from build123d import *

# Parameters (mm, degrees)
F0_W      = 58.45
F0_H      = 12.7
F1_DEPTH  = 2.5
F2_W      = 58.45
F2_H      = 1.21
F6_DEPTH  = 0.6
F4_W      = 58.45
F4_H      = 1.21
F7_DEPTH  = 0.6
F5_W      = 1.21
F5_H      = 12.7
F8_DEPTH  = 0.6
F3_W      = 1.21
F3_H      = 12.7
F9_DEPTH  = 0.6
F10_W     = 3.2
F10_H     = 8.5
F11_DEPTH = 1
F12_R     = 2.4
F14_W     = 4.5
F14_H     = 8.5
F13_W     = 4.5
F13_H     = 8.5
F15_DEPTH = 13.25
F16_R     = 2.24999
F17_R     = 3.15
F18_DEPTH = 16.751


# Not quite as in the source:
# - a fillet or chamfer is up to 0.001 mm smaller than in the source, because OpenCascade refuses the exact size


with BuildPart() as f1:
    # F0 (on Front) → F1 (new body)
    with BuildSketch(Plane.XZ):
        Rectangle(F0_W, F0_H)
    extrude(amount=-F1_DEPTH)

    # F2 (on face) → F6 (cut)
    with BuildSketch(Plane.XY.offset(6.35)):
        with Locations((0, 1.245)):
            Rectangle(F2_W, F2_H)
    extrude(amount=-F6_DEPTH, mode=Mode.SUBTRACT)

    # F4 (on face) → F7 (cut)
    with BuildSketch(Plane(origin=(0, 0, -6.35), x_dir=(1, 0, 0), z_dir=(0, 0, -1))):
        with Locations((0, -1.245)):
            Rectangle(F4_W, F4_H)
    extrude(amount=-F7_DEPTH, mode=Mode.SUBTRACT)

    # F5 (on face) → F8 (cut)
    with BuildSketch(Plane.YZ.offset(29.225)):
        with Locations((1.245, 0)):
            Rectangle(F5_W, F5_H)
    extrude(amount=-F8_DEPTH, mode=Mode.SUBTRACT)

    # F3 (on face) → F9 (cut)
    with BuildSketch(Plane(origin=(-29.225, 0, 0), x_dir=(0, -1, 0), z_dir=(-1, 0, 0))):
        with Locations((-1.245, 0)):
            Rectangle(F3_W, F3_H)
    extrude(amount=-F9_DEPTH, mode=Mode.SUBTRACT)

    # F10 (on face) → F11 (join)
    with BuildSketch(Plane(origin=(0, 2.5, 0), x_dir=(-1, 0, 0), z_dir=(0, 1, 0))):
        with Locations((-27.625, -1.15)):
            Rectangle(F10_W, F10_H)
        with Locations((27.625, -1.15)):
            Rectangle(F10_W, F10_H)
    extrude(amount=F11_DEPTH)

    # F12
    f12_edges = [f1.edges().sort_by_distance(p)[0] for p in [
        (-29.225, 2.175, -6.35),
        (-28.625, 1.245, -5.75),
        (-29.225, 0.32, -6.35),
        (-29.225, 0.32, 6.35),
        (-28.625, 1.245, 5.75),
        (-29.225, 2.175, 6.35),
        (29.225, 0.32, 6.35),
        (28.625, 1.245, 5.75),
        (29.225, 2.175, 6.35),
        (29.225, 0.32, -6.35),
        (28.625, 1.245, -5.75),
        (29.225, 2.175, -6.35),
    ]]
    fillet(f12_edges, radius=F12_R)

    # F14 (on face) + F13 (on face) → F15 (join)
    with BuildSketch(Plane(origin=(0, 3.5, 0), x_dir=(-1, 0, 0), z_dir=(0, 1, 0))):
        with Locations((28.275, -1.15)):
            Rectangle(F14_W, F14_H)
    with BuildSketch(Plane(origin=(0, 3.5, 0), x_dir=(-1, 0, 0), z_dir=(0, 1, 0))):
        with Locations((-28.275, -1.15)):
            Rectangle(F13_W, F13_H)
    extrude(amount=F15_DEPTH)

    # F16 (radius 2.25 in the source; OpenCascade refuses exactly that, so slightly less here)
    f16_edges = [f1.edges().sort_by_distance(p)[0] for p in [
        (26.025, 16.75, -1.15),
        (30.525, 16.75, -1.15),
        (-26.025, 16.75, -1.15),
        (-30.525, 16.75, -1.15),
    ]]
    fillet(f16_edges, radius=F16_R)

    # F17 (on face) → F18 (cut, through all)
    with BuildSketch(Plane.XZ):
        with Locations((19.8096737738, 3.1)):
            Circle(F17_R)
        with Locations((5.8772991731, 3.1)):
            Circle(F17_R)
        with Locations((-7.8854865344, 3.1)):
            Circle(F17_R)
        with Locations((-20.6904198083, 3.1)):
            Circle(F17_R)
    extrude(amount=-F18_DEPTH, mode=Mode.SUBTRACT)


solid = f1.part
Part model, mm, in its own coordinate system. A direction names the side the tool comes from. Coordinates: 2 decimals unless noted, no trailing zeros. Order: outer loops, then holes, each group sorted by start corner. A loop starts at its lowest first (then second) coordinate and runs counter-clockwise, first axis right, second up.
(1) Pin check, flat tips, straight feed: pin 1 Ø3 at (x, y) = (-3.5, 5) entering from -Z; pin 2 Ø1.3 at (x, y) = (-29, 7) entering from +Z; pin 3 Ø0.6 at (x, y) = (-25, 1.5) entering from +Z; pin 4 Ø0.6 at (y, z) = (1.5, -1) entering from +X (3 decimals). Stop position of each tip, or through.
Check sheet entries:
pin 1: passes through
pin 2: stops at z = 3.1
pin 3: stops at z = 5.75
pin 4: stops at x = 28.625
(2) Slice it at D-D, the plane y = 15.25. Write the cut outline in (x, z).
Check sheet entries:
outline: (-30.4, -5.4) - (-26.15, -5.4) - (-26.15, 3.1) - (-30.4, 3.1) - close; (26.15, -5.4) - (30.4, -5.4) - (30.4, 3.1) - (26.15, 3.1) - close
(3) Slice it at A-A, the plane y = 5.5. Write the cut outline in (x, z) (3 decimals), and give its area (3 significant figures).
Check sheet entries:
outline: (-30.525, -5.4) - (-26.025, -5.4) - (-26.025, 3.1) - (-30.525, 3.1) - close; (26.025, -5.4) - (30.525, -5.4) - (30.525, 3.1) - (26.025, 3.1) - close
area: 76.5 mm2
(4) Slice it at C-C, the plane x = 2. Write the cut outline in (y, z), and give its area (3 significant figures).
Check sheet entries:
outline: (0, -6.35) - (0.64, -6.35) - (0.64, -5.75) - (1.85, -5.75) - (1.85, -6.35) - (2.5, -6.35) - (2.5, 6.35) - (1.85, 6.35) - (1.85, 5.75) - (0.64, 5.75) - (0.64, 6.35) - (0, 6.35) - close
area: 30.3 mm2
(5) Tool access for faces 1 (the face through (-28, 10, -5.4)), 2 (the face through (28.625, 1, 0)), 3 (the face through (24, 1, 5.75)): list every direction of +Z, -Z, +X, -X, +Y, -Y with a clear straight run to the whole face (end or side of a thin tool).
Check sheet entries:
face 1: -Z, +X, -X, +Y
face 2: +Z, -Z, +X
face 3: +Z, +X, -X
(6) Probe L1, parallel to X at y = 6, z = 1.75 (3 decimals); L2, parallel to X at y = 2, z = 4.75; L3, parallel to Y at x = 8, z = -2.5. List the from-to ranges inside material, lowest first.
Check sheet entries:
L1: x = -30.525 to -26.025, 26.025 to 30.525
L2: x = -29.09 to -23.37, -18.01 to -10.57, -5.2 to 3.19, 8.56 to 17.13, 22.49 to 29.09
L3: y = 0 to 2.5
(7) Slice it at B-B, the plane x = 19. Write the cut outline in (y, z), and give its area (3 significant figures).
Check sheet entries:
outline: (0, -6.35) - (0.64, -6.35) - (0.64, -5.75) - (1.85, -5.75) - (1.85, -6.35) - (2.5, -6.35) - (2.5, 0.06) - (0, 0.06) - close; (0, 6.14) - (0.64, 6.14) - (0.64, 6.35) - (0, 6.35) - close; (1.85, 6.14) - (2.5, 6.14) - (2.5, 6.35) - (1.85, 6.35) - close
area: 15.6 mm2
(8) Pull direction Y, two halves, no side cores. Call faces 4 (the face through (-24, 1, 5.75)), 5 (the face through (-29.225, 3, 0)), 6 (the face through (30, 3.5, -1)), 7 (the face through (-2, 1.85, -6)): pulls with the +Y half, pulls with the -Y half, needs draft (parallel to the pull), parting line crosses it, or undercut.
Check sheet entries:
face 4: undercut
face 5: needs draft
face 6: pulls with the -Y half
face 7: undercut
